The model under review builds one solid part; all positions refer to its coordinate system, in mm. A direction names the side the tool comes from. Give positions to 0.01 mm unless a question says otherwise; leave off trailing zeros. Loops run counter-clockwise (first coordinate to the right, second up) from the corner with the lowest first, then second, coordinate; pieces in that order, holes last. Notation, with made-up numbers: M 73.25,87 L 81.25,87 A22 ccw 81.25,125 Z; hole C 79.5,-38.5 d3. An arc over 180 degrees is marked long. Write item = value, one per line. Start each with the question number.
1. We need section D-D on x = 10. Give the boundary of the cut face in (y, z), then the cut area to 3 significant figures.
2. We need section C-C on x = -0.25. Give the boundary of the cut face in (y, z).
3. Wall thickness on line 1 along Y through (x, z) = (-1, -1.5); line 2 along X through (y, z) = (-2, -4); line 3 along Y through (x, z) = (1.25, 0): over which ranges is each line inside the solid? List them lowest first. Write a range as from..to.
4. For faces 1 (the face through (-2.5, 0, -2.5)), 2 (the face through (15.5, 1, 3)), 3 (the face through (-2, -1, 0)), 4 (the face through (2, -3, 0)), 5 (the face through (-2.5, 0, 2.5)), list the 3-axis set-ups (+Z, -Z, +X, -X, +Y, -Y) from which the entire face can be reached by the end or side of a thin tool; tool diameter is ignored.
5. For pin 1 (0.8 mm diameter, centred on y = 1.5, z = -0.5, fed in from -X); pin 2 (2 mm diameter, centred on x = 1, z = -2, fed in from -Y); pin 3 (4 mm diameter, centred on x = 14, z = 4, fed in from +Y), all flat-tipped, find the tip position at first contact; note any pin that passes through.
6. We need section A-A on y = 0. Give the boundary of the cut face in (x, z), then the cut area to 3 significant figures.
from build123d import *

# Parameters (mm, degrees)
EXTRUDE_3_DEPTH = 5


with BuildPart() as part:
    # 草图1 → 旋转1 (revolve)
    with BuildSketch(Plane.XY):
        Polygon((0, 0), (0, 2.5), (0.5, 3), (2.5, 3), (2.5, 4.9), (2.6, 5), (5.4, 5), (5.5, 4.9), (5.5, 4), (15.4, 4), (15.5, 3.9), (15.5, 3), (19.5, 3), (20, 2.5), (20, 0), align=None)
    revolve(axis=Axis((20, 0, 0), (-1, 0, 0)))

    # 草图4 → 凸台-拉伸3 (add)
    with BuildSketch(Plane(origin=(0, 0, 0), x_dir=(0, 0, -1), z_dir=(1, 0, 0))):
        with BuildLine():
            Line((0, 1), (2.291287847, 1))
            ThreePointArc((2.291287847, 1), (2.5, 0), (2.291287847, -1))
            Line((2.291287847, -1), (0, -1))
            Line((0, -1), (-2.291287847, -1))
            ThreePointArc((-2.291287847, -1), (-2.5, 0), (-2.291287847, 1))
            Line((-2.291287847, 1), (0, 1))
        make_face()
    extrude(amount=-EXTRUDE_3_DEPTH)


solid = part.part
Final values:
q1.outline = C 0,0 d8
q1.area = 50.3 mm²
q2.outline = M -1,-2.29 A2.5 ccw 1,-2.29 L 1,2.29 A2.5 ccw -1,2.29 Z
q3.line_1 = -1..1
q3.line_2 = 2.5..5.5
q3.line_3 = -3..3
q4.face_1 = -Z, -X
q4.face_2 = +X
q4.face_3 = +Z, -Z, -X, -Y
q4.face_4 = -X
q4.face_5 = +Z, -X
q5.pin_1 = 0
q5.pin_2 = -2.83
q5.pin_3 = 3.46
q6.outline = M -5,-2.5 L 0,-2.5 L 0.5,-3 L 2.5,-3 L 2.5,-4.9 L 2.6,-5 L 5.4,-5 L 5.5,-4.9 L 5.5,-4 L 15.4,-4 L 15.5,-3.9 L 15.5,-3 L 19.5,-3 L 20,-2.5 L 20,2.5 L 19.5,3 L 15.5,3 L 15.5,3.9 L 15.4,4 L 5.5,4 L 5.5,4.9 L 5.4,5 L 2.6,5 L 2.5,4.9 L 2.5,3 L 0.5,3 L 0,2.5 L -5,2.5 Z
q6.area = 176 mm²
